Can you work these out from the drawing? Everything is in mm from the part's minimum corner. Coordinates: 2 decimals unless noted, no trailing zeros. Loops run counter-clockwise (first coordinate to the right, second up) from the corner with the lowest first, then second, coordinate; pieces in that order, holes last. Notation, with made-up numbers: (81, 1.25) -> (110, 1.25) arc R26 cw to (110, 24.25) -> close; hole circle Ø8 at (-30.75, -10.75). An arc over 180 degrees is marked (long way). Use one line per item in the form item = value. Start each with the question number.
(1) Imagine slicing it at C-C (z = 30.5). List the corners of the cut face in (x, y) for me, plus the area to 3 significant figures.
(2) Imagine slicing it at D-D (x = 37). State how many separate pieces and enclosed holes the cut face has, plus the area to 3 significant figures.
(3) I need wall thicknesses on line 1 (Z direction, x = 21.5, y = 39.5); line 2 (Y direction, x = 2, z = 29); line 3 (Y direction, x = 26, z = 3). Which ranges of each line are inside material? Lowest first, please. Write a range as [from, to].
(4) Imagine slicing it at A-A (x = 25). List the corners of the cut face in (y, z) for me, plus the area to 3 significant figures.
(5) Imagine slicing it at B-B (y = 25). List the corners of the cut face in (x, z) for me, plus the area to 3 significant figures.
(6) I'm going to push flat-ended pins straight in: pin 1 (2 mm diameter, centred on y = 25, z = 44.5, fed in from +X); pin 2 (2 mm diameter, centred on x = 5, z = 13, fed in from -Y); pin 3 (8 mm diameter, centred on x = 42, z = 31, fed in from +Y). Where does each tip first touch, or does it pass through?
(7) Thinking about a two-plate mould opening in Z: for the marked faces 1, 2 and 3, which applies, released by +Z, released by -Z, zero draft, split by the parting line, or undercut?
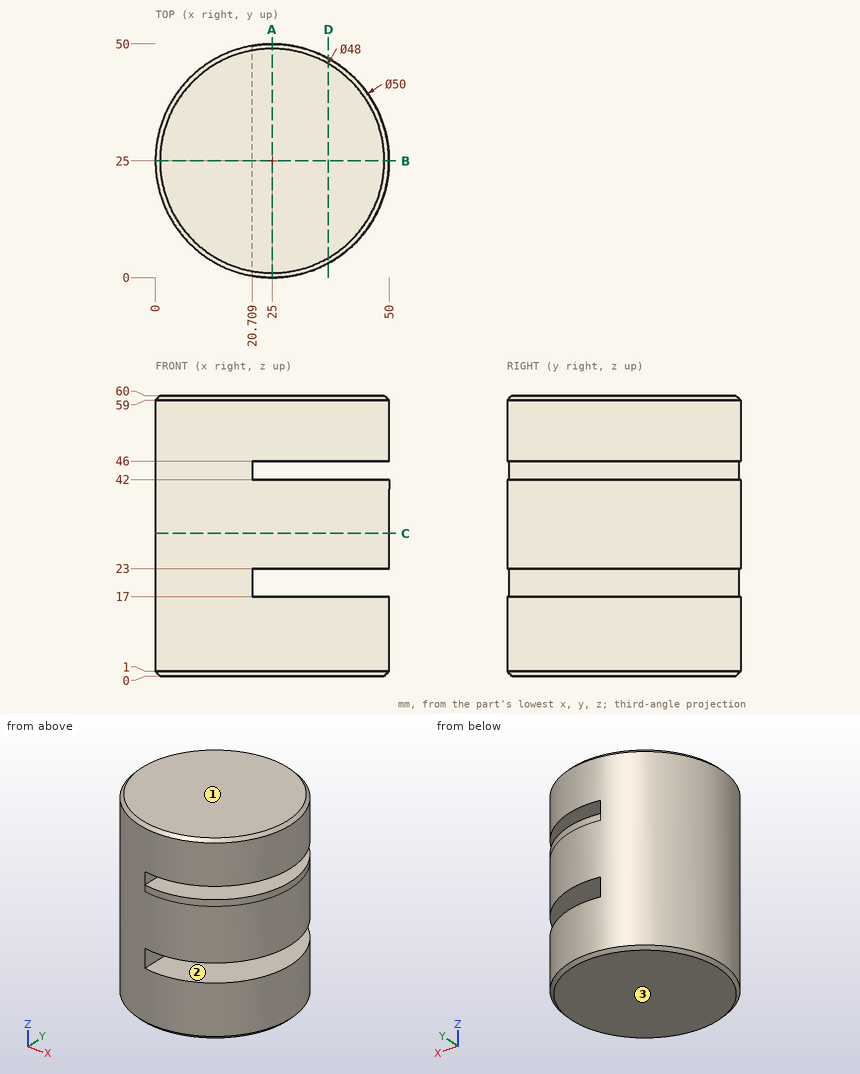
Worked out:
q1.outline = circle Ø50 at (25, 25)
q1.area = 1,960 mm2
q2.separate_pieces = 3
q2.enclosed_holes = 0
q2.area = 2,190 mm2
q3.line_1 = [0, 17], [23, 42], [46, 60]
q3.line_2 = [15.2, 34.8]
q3.line_3 = [0.02, 49.98]
q4.outline = (0, 1) -> (1, 0) -> (49, 0) -> (50, 1) -> (50, 17) -> (0, 17) -> close; (0, 23) -> (50, 23) -> (50, 42) -> (0, 42) -> close; (0, 46) -> (50, 46) -> (50, 59) -> (49, 60) -> (1, 60) -> (0, 59) -> close
q4.area = 2,500 mm2
q5.outline = (0, 1) -> (1, 0) -> (49, 0) -> (50, 1) -> (50, 17) -> (20.71, 17) -> (20.71, 23) -> (50, 23) -> (50, 42) -> (20.71, 42) -> (20.71, 46) -> (50, 46) -> (50, 59) -> (49, 60) -> (1, 60) -> (0, 59) -> close
q5.area = 2,710 mm2
q6.pin_1 = 20.71
q6.pin_2 = 8.75
q6.pin_3 = 46.35
q7.face_1 = released by +Z
q7.face_2 = undercut
q7.face_3 = released by -Z
